Geometry: final body of the model. Coordinates: model frame, mm. A direction names the side the tool comes from. Give positions to 0.01 mm unless a question says otherwise; leave off trailing zeros. Write each loop counter-clockwise with the first axis right and the second up, starting at its lowest first coordinate (ties: lowest second). Pieces come first, ordered by that corner, then holes. Notation, with made-up numbers: (-3, -39.75) -> (12, -39.75) arc R6 ccw to (12, -35.75) -> close; hole circle Ø10 at (78, 59). An arc over 180 degrees is marked (long way). Use CSV: the item, a comma, the result in double quotes. Start each with the question number.
1) Contact query for flat-ended pins moving along their axis: P1, Ø6, axis at x = -7.5, z = 3, coming from the +Y side; P2, Ø1.5, axis at x = -20.5, z = 4, coming from the -Y side; P3, Ø1.5, axis at y = 2, z = 7.5, coming from the -X side. Output: stop coordinate, or through.
2) Set-up query: faces 4 (the face through (12, 22, 5)), 5 (the face through (-6, 22, 5)), 6 (the face through (-1, 0, 10)), 7 (the face through (8.488, 27.241, 4.93)). Return all of +Z, -Z, +X, -X, +Y, -Y with unobstructed straight access to the full face (end or side cutting, diameter ignored); none if empty.
3) Section A-A (z = 2.75). Output: boundary loops of the cut face in (x, y).
4) Section C-C (x = 0). Output: boundary loops of the cut face in (y, z), plus the area to 3 significant figures.
5) Section B-B (y = -22). Output: boundary loops of the cut face in (x, z).
6) Draft query along Y for faces 1 (the face through (17.2, 21.475, 4.93)), 2 (the face through (-1, 0, 0)), 3 (the face through (20.11, 1.475, 4.93)). Return one class per face: pulls with the +Y half, pulls with the -Y half, needs draft (parallel to the pull), parting line crosses it, or undercut.
7) Material intervals for line 1 (X direction, y = 5, z = 6.5); line 2 (Y direction, x = 17, z = 2.5); line 3 (Y direction, x = -22.5, z = 4.25), sorted ascending. Write a range as [from, to].
```python
from build123d import *

# Parameters (mm, degrees)
BOX002_W                  = 10
BOX002_H                  = 14
BOX002_DEPTH              = 15
CYLINDER002_R             = 5
CYLINDER002_DEPTH         = 15
CYLINDER001_R             = 5
CYLINDER001_DEPTH         = 15
CYLINDER004_R             = 4
CYLINDER004_DEPTH         = 15
CYLINDER003_R             = 5
CYLINDER003_DEPTH         = 15
FUSION003_PLACEMENT_ANGLE = 20
BOX001_W                  = 6
BOX001_H                  = 25
BOX001_DEPTH              = 38
BOX001_PLACEMENT_ANGLE    = -17
BOX_W                     = 59
BOX_H                     = 14
BOX_DEPTH                 = 15
CYLINDER_R                = 30
CYLINDER_DEPTH            = 10
FILLET_R                  = 20
FILLET001_R               = 15
FILLET002_R               = 4
FILLET003_R               = 3


with BuildPart() as cube002:
    # Box002 → Box002 (new body)
    with BuildSketch(Plane(origin=(23, -9, -2), x_dir=(1, 0, 0), z_dir=(0, 0, 1))):
        with Locations((5, 7)):
            Rectangle(BOX002_W, BOX002_H)
    extrude(amount=BOX002_DEPTH)


with BuildPart() as fusion:
    # Cylinder002 → Cylinder002 (new body)
    with BuildSketch(Plane(origin=(24, 2, -3), x_dir=(1, 0, 0), z_dir=(0, 0, 1))):
        Circle(CYLINDER002_R)
    extrude(amount=CYLINDER002_DEPTH)

    # Fusion: union Cube002
    add(cube002.part)


with BuildPart() as fusion001:
    # Cylinder001 → Cylinder001 (new body)
    with BuildSketch(Plane(origin=(29, 8, -3), x_dir=(1, 0, 0), z_dir=(0, 0, 1))):
        Circle(CYLINDER001_R)
    extrude(amount=CYLINDER001_DEPTH)

    # Fusion001: union Fusion
    add(fusion.part)


with BuildPart() as fusion002:
    # Cylinder004 → Cylinder004 (new body)
    with BuildSketch(Plane(origin=(26, -11, -3), x_dir=(1, 0, 0), z_dir=(0, 0, 1))):
        Circle(CYLINDER004_R)
    extrude(amount=CYLINDER004_DEPTH)

    # Fusion002: union Fusion001
    add(fusion001.part)


with BuildPart() as fusion003:
    # Cylinder003 → Cylinder003 (new body)
    with BuildSketch(Plane(origin=(23, -5, -3), x_dir=(1, 0, 0), z_dir=(0, 0, 1))):
        Circle(CYLINDER003_R)
    extrude(amount=CYLINDER003_DEPTH)

    # Fusion003: union Fusion002
    add(fusion002.part)


with BuildPart() as fusion003_1:
    # Fusion003 placement: moved
    add(fusion003.part.moved(Location((1, 1, 0))).rotate(Axis((1, 1, 0), (0, 0, 1)), FUSION003_PLACEMENT_ANGLE))


with BuildPart() as cube001:
    # Box001 → Box001 (new body)
    with BuildSketch(Plane.XY):
        with Locations((3, 12.5)):
            Rectangle(BOX001_W, BOX001_H)
    extrude(amount=BOX001_DEPTH)


with BuildPart() as cube001_1:
    # Box001 placement: moved
    add(cube001.part.moved(Location((0, 20, -14))).rotate(Axis((0, 20, -14), (0, 0, 1)), BOX001_PLACEMENT_ANGLE))


with BuildPart() as cut:
    # Box → Box (new body)
    with BuildSketch(Plane(origin=(-29, 22, -3), x_dir=(1, 0, 0), z_dir=(0, 0, 1))):
        with Locations((29.5, 7)):
            Rectangle(BOX_W, BOX_H)
    extrude(amount=BOX_DEPTH)

    # Cut: cut Cube001
    add(cube001_1.part, mode=Mode.SUBTRACT)


with BuildPart() as cut002:
    # Cylinder → Cylinder (new body)
    with BuildSketch(Plane.XY):
        Circle(CYLINDER_R)
    extrude(amount=CYLINDER_DEPTH)

    # Cut001: cut Cut
    add(cut.part, mode=Mode.SUBTRACT)

    # Fillet
    fillet_edges = [cut002.edges().sort_by_distance(p)[0] for p in [
        (-20.396078, 22, 5),
    ]]
    fillet(fillet_edges, radius=FILLET_R)

    # Fillet001
    fillet001_edges = [cut002.edges().sort_by_distance(p)[0] for p in [
        (20.396078, 22, 5),
    ]]
    fillet(fillet001_edges, radius=FILLET001_R)

    # Fillet002
    fillet002_edges = [cut002.edges().sort_by_distance(p)[0] for p in [
        (0.611461, 22, 5),
    ]]
    fillet(fillet002_edges, radius=FILLET002_R)

    # Fillet003
    fillet003_edges = [cut002.edges().sort_by_distance(p)[0] for p in [
        (6.885612, 22, 5),
    ]]
    fillet(fillet003_edges, radius=FILLET003_R)

    # Cut002: cut Fusion003
    add(fusion003_1.part, mode=Mode.SUBTRACT)


solid = cut002.part
```
Answers follow:
1,P1,"stops at y = 22"
1,P2,"stops at y = -22.58"
1,P3,"stops at x = -29.97"
2,face 4,"+Z, -Z, +X, +Y"
2,face 5,"+Z, -Z, -X, +Y"
2,face 6,"+Z, +X, -X, +Y, -Y"
2,face 7,"+Z, -Z, +X"
3,outline,"(-29.39, 6) arc R30 ccw (long way) to (29.67, -4.42) arc R4 cw to (25.21, -0.75) arc R5 cw to (20.14, 6.9) arc R5 cw to (21.25, 15.82) arc R5 cw to (20.76, 19.99) arc R15 ccw to (13.27, 22) -> (10.94, 22) arc R3 cw to (8.07, 25.88) -> (8.92, 28.64) arc R30 ccw to (3.01, 29.85) -> (1.48, 24.83) arc R4 cw to (-2.35, 22) -> (-9.8, 22) arc R20 ccw to start"
4,outline,"(-30, 0) -> (22.76, 0) -> (22.76, 10) -> (-30, 10) -> close"
4,area,"528 mm^2"
5,outline,"(-20.4, 0) -> (20.4, 0) -> (20.4, 10) -> (-20.4, 10) -> close"
6,face 1,"pulls with the +Y half"
6,face 2,"needs draft"
6,face 3,"undercut"
7,line 1,"x = [-29.58, 19.39]"
7,line 2,"y = [-24.72, 21.53]"
7,line 3,"y = [-19.84, 17.45]"
